from build123d import *

# Parameters (mm, degrees)
SKETCH1_W           = 80.20256146
SKETCH1_H           = 63.780997334
SKETCH1_R           = 1.5
SKETCH1_W_2         = 15.405665538
SKETCH1_H_2         = 22.140498667
SKETCH1_W_3         = 11.853085899
SKETCH1_W_4         = 26.943810023
BOSS_EXTRUDE1_DEPTH = 1.5


with BuildPart() as part:
    # Sketch1 → Boss-Extrude1 (new, symmetric)
    with BuildSketch(Plane(origin=(0, 0, 0), x_dir=(1, 0, 0), z_dir=(0, 1, 0))):
        Rectangle(SKETCH1_W, SKETCH1_H)
        with Locations(Location((-21.864035064, 0, 0), (0, 0, 270))):
            Circle(SKETCH1_R, mode=Mode.SUBTRACT)
        with Locations(Location((-1.864035064, 0, 0), (0, 0, 270))):
            Circle(SKETCH1_R, mode=Mode.SUBTRACT)
        with Locations(Location((25.635964936, 0, 0), (0, 0, 270))):
            Circle(SKETCH1_R, mode=Mode.SUBTRACT)
        with Locations((-25.898447961, -14.320249334)):
            Rectangle(SKETCH1_W_2, SKETCH1_H_2, mode=Mode.SUBTRACT)
        with Locations((-25.898447961, 14.320249334)):
            Rectangle(SKETCH1_W_2, SKETCH1_H_2, mode=Mode.SUBTRACT)
        with Locations((27.674737781, -14.320249334)):
            Rectangle(SKETCH1_W_3, SKETCH1_H_2, mode=Mode.SUBTRACT)
        with Locations((1.77628982, 14.320249334)):
            Rectangle(SKETCH1_W_4, SKETCH1_H_2, mode=Mode.SUBTRACT)
        with Locations((27.674737781, 14.320249334)):
            Rectangle(SKETCH1_W_3, SKETCH1_H_2, mode=Mode.SUBTRACT)
        with Locations((1.77628982, -14.320249334)):
            Rectangle(SKETCH1_W_4, SKETCH1_H_2, mode=Mode.SUBTRACT)
    extrude(amount=BOSS_EXTRUDE1_DEPTH, both=True)


solid = part.part
Can you work these out from the model? Positions are in its coordinate system, mm. A direction names the side the tool comes from. Give positions to 0.01 mm unless a question says otherwise; leave off trailing zeros. Loops run counter-clockwise (first coordinate to the right, second up) from the corner with the lowest first, then second, coordinate; pieces in that order, holes last. Notation, with made-up numbers: M 74,43 L 80,43 A34 ccw 80,78 Z; hole C 24,7.5 d8. An arc over 180 degrees is marked long. One line per item, written item: value.
1) On a 3-axis mill with a long thin cutter (end or side, diameter ignored), from which of +Z, -Z, +X, -X, +Y, -Y can I reach the whole of each face in a straight line? I mean faces 1 (the face through (-40.101, 0, 0)), 2 (the face through (28, 0, -25.39)). Say none if no direction works.
Geometry check:
face 1: +Z, -Z, -X, +Y, -Y
face 2: +Y, -Y
2) Please list where these lines run through material, in increasing order: line 1 (X direction, y = 0.4, z = 0); line 2 (X direction, y = -0.6, z = 23); line 3 (Z direction, x = -20, y = -0.9).
Geometry check:
line 1: x = -40.1 to -23.36, -20.36 to -3.36, -0.36 to 24.14, 27.14 to 40.1
line 2: x = -40.1 to -33.6, -18.2 to -11.7, 15.25 to 21.75, 33.6 to 40.1
line 3: z = -31.89 to -25.39, -3.25 to 3.25, 25.39 to 31.89
3) Imagine slicing it at A-A on z = 0. Write out the boundary of the cut face in (x, y), and give its area (3 significant figures).
Geometry check:
outline: M -40.1,-1.5 L -23.36,-1.5 L -23.36,1.5 L -40.1,1.5 Z; M -20.36,-1.5 L -3.36,-1.5 L -3.36,1.5 L -20.36,1.5 Z; M -0.36,-1.5 L 24.14,-1.5 L 24.14,1.5 L -0.36,1.5 Z; M 27.14,-1.5 L 40.1,-1.5 L 40.1,1.5 L 27.14,1.5 Z
area: 214 mm²
4) Thinking about a two-plate mould opening in X: for faces 3 (the face through (8, 1.5, 0)), 4 (the face through (-11.696, 0, 14)), 5 (the face through (40.101, 0, 0)), which applies, +X half, -X half, draft (parallel to the pull), parting line (faces both ways), or undercut?
Geometry check:
face 3: draft
face 4: undercut
face 5: +X half
5) Imagine slicing it at B-B on x = 10. Write out the boundary of the cut face in (y, z).
Geometry check:
outline: M -1.5,-31.89 L 1.5,-31.89 L 1.5,-25.39 L -1.5,-25.39 Z; M -1.5,-3.25 L 1.5,-3.25 L 1.5,3.25 L -1.5,3.25 Z; M -1.5,25.39 L 1.5,25.39 L 1.5,31.89 L -1.5,31.89 Z
6) Imagine slicing it at C-C on y = -1. Count the separate pieces of the cut face and the enclosed holes in it, and give its area (3 significant figures).
Geometry check:
separate pieces: 1
enclosed holes: 9
area: 2,690 mm²
7) I'm going to push flat-ended pins straight in: pin 1 (12 mm diameter, centred on x = -8.5, z = 3.5, fed in from +Y); pin 2 (1 mm diameter, centred on x = -20.5, z = -18.5, fed in from +Y). Where does each tip first touch, or does it pass through?
Geometry check:
pin 1: stops at y = 1.5
pin 2: passes through
